Part print with two shaded views. Sizes in mm from the minimum x, y, z corner. A direction names the side the tool comes from. Coordinates: 2 decimals unless noted, no trailing zeros. Loops run counter-clockwise (first coordinate to the right, second up) from the corner with the lowest first, then second, coordinate; pieces in that order, holes last.
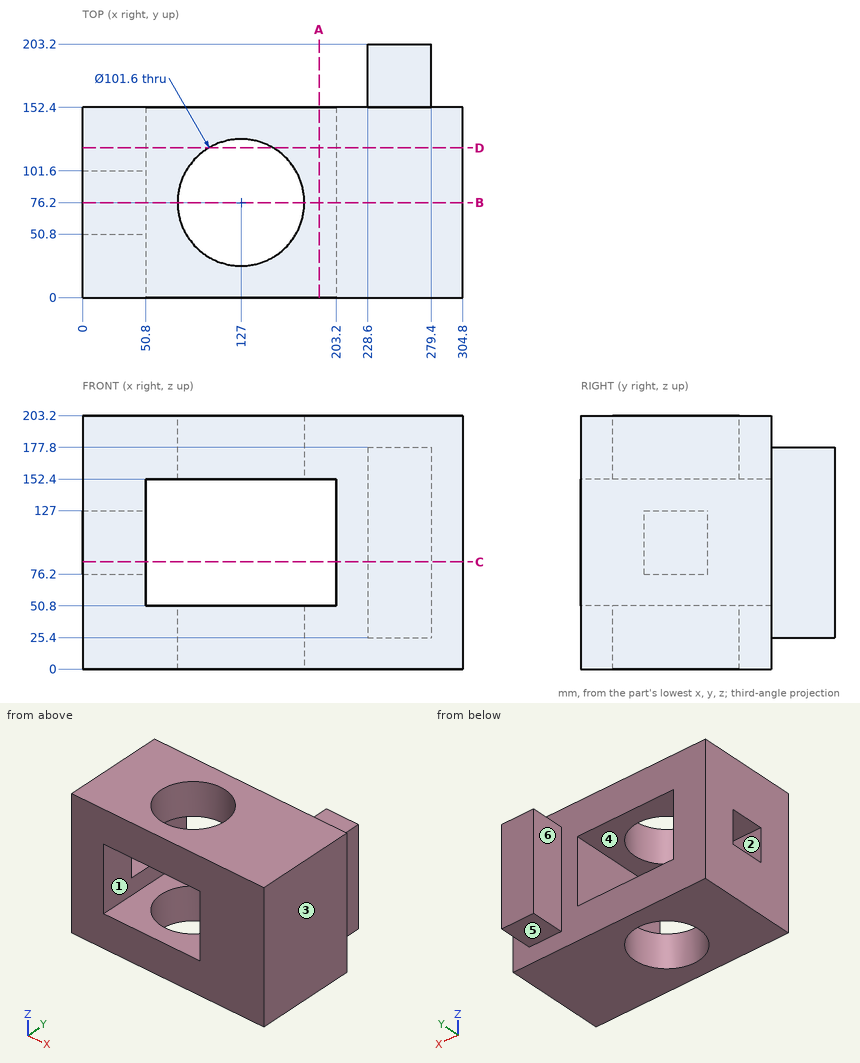
Q1. Slice it at D-D (y = 120). List the corners of the cut face in (x, z), and give its area (3 significant figures).
Answers:
outline: (0, 0) - (101.27, 0) - (101.27, 50.8) - (50.8, 50.8) - (50.8, 152.4) - (101.27, 152.4) - (101.27, 203.2) - (0, 203.2) - close; (152.73, 0) - (304.8, 0) - (304.8, 203.2) - (152.73, 203.2) - (152.73, 152.4) - (203.2, 152.4) - (203.2, 50.8) - (152.73, 50.8) - close
area: 41,200 mm2
Q2. Slice it at A-A (x = 189.5). List the corners of the cut face in (y, z).
Answers:
outline: (0, 0) - (152.4, 0) - (152.4, 50.8) - (0, 50.8) - close; (0, 152.4) - (152.4, 152.4) - (152.4, 203.2) - (0, 203.2) - close
Q3. Slice it at C-C (z = 86). List the corners of the cut face in (x, y), and give its area (3 significant figures).
Answers:
outline: (0, 0) - (50.8, 0) - (50.8, 50.8) - (0, 50.8) - close; (0, 101.6) - (50.8, 101.6) - (50.8, 152.4) - (0, 152.4) - close; (203.2, 0) - (304.8, 0) - (304.8, 152.4) - (279.4, 152.4) - (279.4, 203.2) - (228.6, 203.2) - (228.6, 152.4) - (203.2, 152.4) - close
area: 23,200 mm2
Q4. Slice it at B-B (y = 76.2). List the corners of the cut face in (x, z), and give its area (3 significant figures).
Answers:
outline: (0, 0) - (76.2, 0) - (76.2, 50.8) - (50.8, 50.8) - (50.8, 76.2) - (0, 76.2) - close; (0, 127) - (50.8, 127) - (50.8, 152.4) - (76.2, 152.4) - (76.2, 203.2) - (0, 203.2) - close; (177.8, 0) - (304.8, 0) - (304.8, 203.2) - (177.8, 203.2) - (177.8, 152.4) - (203.2, 152.4) - (203.2, 50.8) - (177.8, 50.8) - close
area: 33,500 mm2
Q5. Mould opens along X. For the marked faces 1, 2 and 3 say: +X half, -X half, draft (parallel to the pull), parting line (faces both ways), or undercut.
Answers:
face 1: undercut
face 2: draft
face 3: +X half
Q6. Drill centre lines: line 1 (X direction, y = 76, z = 22); line 2 (X direction, y = 96.5, z = 140); line 3 (Y direction, x = 127, z = 37). Where is each one in solid material? Low to high.
Answers:
line 1: x = 0 to 76.2, 177.8 to 304.8
line 2: x = 0 to 50.8, 203.2 to 304.8
line 3: y = 0 to 25.4, 127 to 152.4
Q7. Flat gauge pin, fed straight in: P1, Ø5, axis at x = 46, z = 79.5, coming from the +Y side. Where does the tip first touch, or does it go through?
Answers:
P1: stops at y = 152.4
Q8. Which spindle directions (+Z, -Z, +X, -X, +Y, -Y) get a long thin tool onto all of the face, cutting with end or side? Do the marked faces 4, 5 and 6. Say none if no direction does.
Answers:
face 4: +Y, -Y
face 5: -Z, +X, -X, +Y
face 6: +Z, -Z, -X, +Y
